```python
from build123d import *

# Parameters (mm, degrees)
SKETCH1_W           = 394.926652775
SKETCH1_H           = 202.769674437
BOSS_EXTRUDE1_DEPTH = 333
SHELL5_T            = -10
BOSS_EXTRUDE2_DEPTH = 7
SKETCH19_R          = 24.92303726
CUT_EXTRUDE1_DEPTH  = 14
BOSS_EXTRUDE3_DEPTH = 7
SKETCH23_R          = 24.92303726
CUT_EXTRUDE2_DEPTH  = 14
SKETCH24_W          = 378.549978472
SKETCH24_H          = 14.5311901
CUT_EXTRUDE6_DEPTH  = 30
SKETCH25_W          = 25.994787148
SKETCH25_H          = 10.885886146
BOSS_EXTRUDE5_DEPTH = 14
SKETCH27_W          = 29.478735589
SKETCH27_H          = 14.140745891
BOSS_EXTRUDE7_DEPTH = 14
EXTRUDE_THIN2_REACH = 553.377
SKETCH33_W          = 10
SKETCH33_H          = 122.071459974
CUT_EXTRUDE8_DEPTH  = 49
SKETCH35_W          = 10
SKETCH35_H          = 10.654236951
CUT_EXTRUDE11_DEPTH = 182.769674437


with BuildPart() as part:
    # Sketch1 → Boss-Extrude1 (new body)
    with BuildSketch(Plane.XY):
        with Locations((197.463326388, 101.384837219)):
            Rectangle(SKETCH1_W, SKETCH1_H)
    extrude(amount=BOSS_EXTRUDE1_DEPTH)

    # Shell5
    shell5_openings = [part.faces().sort_by_distance(p)[0] for p in [
        (197.463326387, 101.384837219, 333),
    ]]
    offset(amount=SHELL5_T, openings=shell5_openings, kind=Kind.INTERSECTION)

    # Sketch18 → Boss-Extrude2 (add, symmetric)
    with BuildSketch(Plane.XY.offset(166.5)):
        with BuildLine():
            Line((10, 128.355944405), (81.814439739, 128.355944405))
            ThreePointArc((81.814439739, 128.355944405), (117.012291579, 93.158092565), (81.814439739, 57.960240724))
            Line((81.814439739, 57.960240724), (10, 57.960240724))
            Line((10, 57.960240724), (10, 128.355944405))
        make_face()
    extrude(amount=BOSS_EXTRUDE2_DEPTH, both=True)

    # Sketch19 → Cut-Extrude1 (cut)
    with BuildSketch(Plane.XY.offset(173.5)):
        with Locations((81.814439739, 93.158092565)):
            Circle(SKETCH19_R)
    extrude(amount=-CUT_EXTRUDE1_DEPTH, mode=Mode.SUBTRACT)

    # Sketch22 → Boss-Extrude3 (add, symmetric)
    with BuildSketch(Plane.XY.offset(166.5)):
        with BuildLine():
            Line((384.926652775, 128.355944405), (291.108955259, 128.355944405))
            ThreePointArc((291.108955259, 128.355944405), (256.621992249, 93.868981396), (291.108955259, 59.382018386))
            Line((291.108955259, 59.382018386), (384.926652775, 59.382018386))
            Line((384.926652775, 59.382018386), (384.926652775, 128.355944405))
        make_face()
    extrude(amount=BOSS_EXTRUDE3_DEPTH, both=True)

    # Sketch23 → Cut-Extrude2 (cut)
    with BuildSketch(Plane.XY.offset(173.5)):
        with Locations((291.108955259, 93.868981396)):
            Circle(SKETCH23_R)
    extrude(amount=-CUT_EXTRUDE2_DEPTH, mode=Mode.SUBTRACT)

    # Sketch24 → Cut-Extrude6 (cut)
    with BuildSketch(Plane(origin=(0, 202.769674437, 0), x_dir=(1, 0, 0), z_dir=(0, 1, 0))):
        with Locations((196.17510715, -13.388641901)):
            Rectangle(SKETCH24_W, SKETCH24_H)
    extrude(amount=-CUT_EXTRUDE6_DEPTH, mode=Mode.SUBTRACT)

    # Sketch25 → Boss-Extrude5 (add)
    with BuildSketch(Plane(origin=(0, 10, 0), x_dir=(1, 0, 0), z_dir=(0, 1, 0))):
        with Locations((19.897511488, -26.097180024)):
            Rectangle(SKETCH25_W, SKETCH25_H)
    extrude(amount=BOSS_EXTRUDE5_DEPTH)

    # Sketch27 → Boss-Extrude7 (add)
    with BuildSketch(Plane(origin=(0, 10, 0), x_dir=(1, 0, 0), z_dir=(0, 1, 0))):
        with Locations((370.710728592, -27.724609897)):
            Rectangle(SKETCH27_W, SKETCH27_H)
    extrude(amount=BOSS_EXTRUDE7_DEPTH)

    # Sketch33 → Extrude-Thin2 (add, up to next)
    with BuildSketch(Plane.XZ.offset(-192.769674437), mode=Mode.PRIVATE) as extrude_thin2_sk1:
        with Locations((202.463326387, 71.035729987)):
            Rectangle(SKETCH33_W, SKETCH33_H)
    extrude_thin2_tool1 = extrude(extrude_thin2_sk1.sketch, amount=EXTRUDE_THIN2_REACH, mode=Mode.PRIVATE) - part.part
    add(extrude_thin2_tool1.solids().sort_by_distance((202.463326, 192.769674, 71.03573))[0])

    # Sketch34 → Cut-Extrude8 (cut)
    with BuildSketch(Plane.ZY.offset(-197.463326387)):
        Polygon((132.071459974, 58.157894262), (39.515170412, 10), (132.071459974, 10), align=None)
    extrude(amount=-CUT_EXTRUDE8_DEPTH, mode=Mode.SUBTRACT)

    # Sketch35 → Cut-Extrude11 (cut)
    with BuildSketch(Plane(origin=(0, 192.769674437, 0), x_dir=(1, 0, 0), z_dir=(0, 1, 0))):
        with Locations((202.463326387, -15.327118476)):
            Rectangle(SKETCH35_W, SKETCH35_H)
    extrude(amount=-CUT_EXTRUDE11_DEPTH, mode=Mode.SUBTRACT)


solid = part.part
```
Part model, mm, in its own coordinate system. A direction names the side the tool comes from. Round coordinates to 2 decimals unless told otherwise and drop trailing zeros. Loops run counter-clockwise (first coordinate to the right, second up) from the corner with the lowest first, then second, coordinate; pieces in that order, holes last.
Item 1: 3-axis set-ups, long thin cutter, end or side, ignore diameter. For faces 1 (the face through (195, 202.77, 164)), 2 (the face through (194, 188, 6.123)), 3 (the face through (195, 103, 0)), 4 (the face through (52, 94, 159.5)), 5 (the face through (202.393, 34.416, 86.441)): which of +Z, -Z, +X, -X, +Y, -Y reach the whole face in a straight line?
Item 2: Drill centre lines: line 1 (X direction, y = 113, z = 115); line 2 (X direction, y = 34, z = 122.5); line 3 (Y direction, x = 54.5, z = 250). Where is each one in solid material? Low to high.
Item 3: Cut at C-C, the plane z = 246. Give the cut face in (x, y).
Item 4: Cut at D-D, the plane x = 184.5. Give the cut face in (y, z).
Item 5: Mould opens along Y. For faces 6 (the face through (32.895, 17, 26)), 7 (the face through (182, 4, 333)), 8 (the face through (46, 57.96, 167)), 9 (the face through (195, 0, 164)) say: +Y half, -Y half, draft (parallel to the pull), parting line (faces both ways), or undercut.
Item 6: Cut at A-A, the plane x = 335. Give the cut face in (y, z).
Item 7: Drop flat-ended pins along their axis: P1, Ø8, axis at x = 203.5, y = 140, coming from the +Z side; P2, Ø8, axis at x = 148.5, y = 50.5, coming from the +Z side; P3, Ø7, axis at x = 17, y = 18, coming from the +Z side. Give the stop position or say it passes through.
Item 8: Cut at B-B, the plane y = 182. Give the cut face in (x, z), then the cut area to 3 significant figures.
A:
1. face 1: +Z, -Z, +X, -X, +Y
1. face 2: +Y
1. face 3: -Z, +X, -X, +Y, -Y
1. face 4: none
1. face 5: +Z
2. line 1: x = 0 to 10, 197.46 to 207.46, 384.93 to 394.93
2. line 2: x = 0 to 10, 384.93 to 394.93
2. line 3: y = 0 to 10, 192.77 to 202.77
3. outline: (0, 0) - (394.93, 0) - (394.93, 202.77) - (0, 202.77) - close; hole (10, 10) - (384.93, 10) - (384.93, 192.77) - (10, 192.77) - close
4. outline: (0, 0) - (202.77, 0) - (202.77, 6.12) - (172.77, 6.12) - (172.77, 10) - (10, 10) - (10, 333) - (0, 333) - close; (192.77, 20.65) - (202.77, 20.65) - (202.77, 333) - (192.77, 333) - close
5. face 6: undercut
5. face 7: draft
5. face 8: undercut
5. face 9: -Y half
6. outline: (0, 0) - (202.77, 0) - (202.77, 6.12) - (172.77, 6.12) - (172.77, 10) - (10, 10) - (10, 333) - (0, 333) - close; (59.38, 159.5) - (128.36, 159.5) - (128.36, 173.5) - (59.38, 173.5) - close; (192.77, 20.65) - (202.77, 20.65) - (202.77, 333) - (192.77, 333) - close
7. P1: stops at z = 132.07
7. P2: stops at z = 10
7. P3: stops at z = 31.54
8. outline: (0, 0) - (394.93, 0) - (394.93, 333) - (384.93, 333) - (384.93, 20.65) - (385.45, 20.65) - (385.45, 6.12) - (6.9, 6.12) - (6.9, 20.65) - (10, 20.65) - (10, 333) - (0, 333) - close; (197.46, 20.65) - (207.46, 20.65) - (207.46, 132.07) - (197.46, 132.07) - close
8. area: 10,000 mm2
